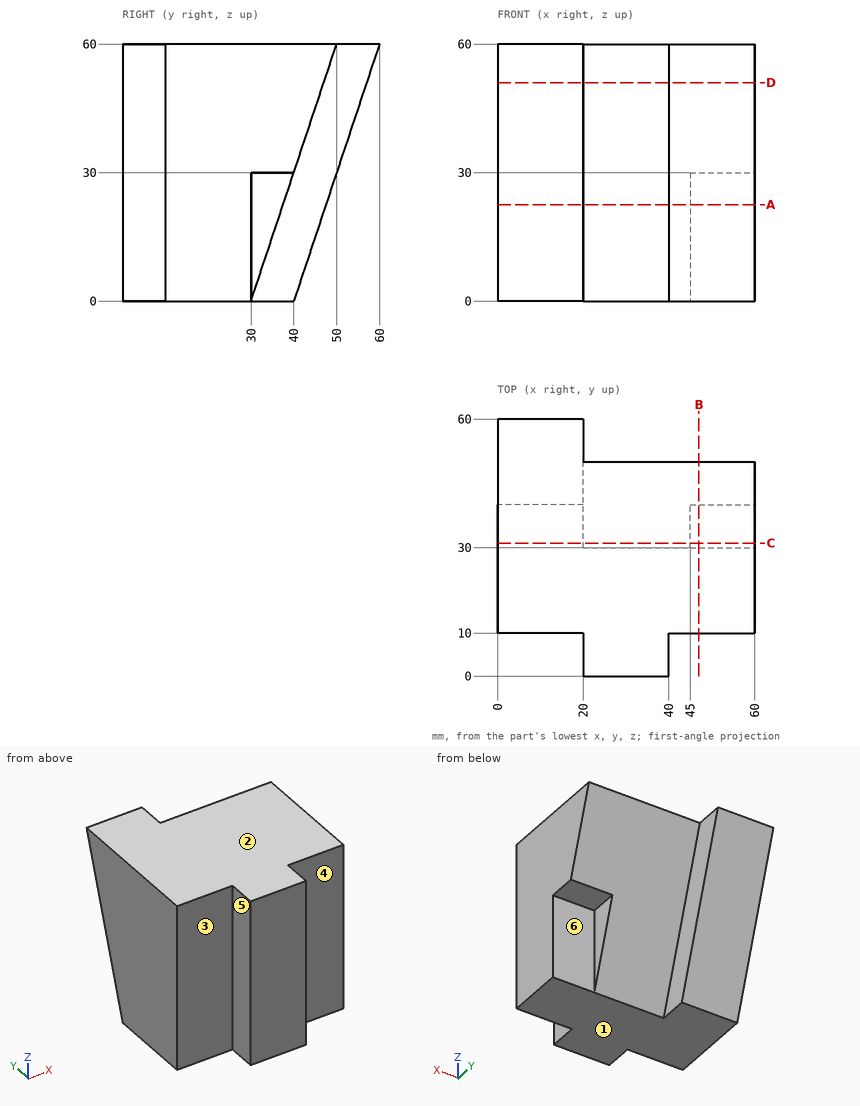
Design review of the part shown in the three views and the two pictorial views. Dimensions are in mm from the part's minimum x, y and z. A direction names the side the tool comes from. Coordinates: 2 decimals unless noted, no trailing zeros. Loops run counter-clockwise (first coordinate to the right, second up) from the corner with the lowest first, then second, coordinate; pieces in that order, holes last.
(1) Consider section C-C, the plane y = 31. Give the boundary of the cut face in (x, z).
Determined:
outline: (0, 0) - (20, 0) - (20, 3) - (45, 3) - (45, 30) - (60, 30) - (60, 60) - (0, 60) - close
(2) Draft analysis for pull direction Z (two halves, no side actions). For the marked faces 1, 2 and 3, state which applies: +Z half, -Z half, draft (parallel to the pull), parting line (faces both ways), or undercut.
Determined:
face 1: -Z half
face 2: +Z half
face 3: draft
(3) Insertion check: P1, Ø2, axis at x = 15.5, z = 26, coming from the -Y side; P2, Ø11, axis at y = 36, z = 12, coming from the +X side; P3, Ø9, axis at y = 46.5, z = 21, coming from the +X side. Each pin has a flat end and moves straight along its axis. Give the tip position at first contact, or say it passes through.
Determined:
P1: stops at y = 10
P2: stops at x = 45
P3: stops at x = 20
(4) Wall thickness on L1, parallel to Y at x = 58.5, z = 21.5; L2, parallel to X at y = 36.5, z = 15; L3, parallel to Y at x = 32.5, z = 46: over which ranges is each line inside the solid? List them lowest first.
Determined:
L1: y = 10 to 30
L2: x = 0 to 20
L3: y = 0 to 45.33
(5) Consider section B-B, the plane x = 47. Give the boundary of the cut face in (y, z), plus the area to 3 significant figures.
Determined:
outline: (10, 0) - (30, 0) - (30, 30) - (40, 30) - (50, 60) - (10, 60) - close
area: 1,650 mm2
(6) Consider section A-A, the plane z = 22.5. Give the boundary of the cut face in (x, y), plus the area to 3 significant figures.
Determined:
outline: (0, 10) - (20, 10) - (20, 0) - (40, 0) - (40, 10) - (60, 10) - (60, 30) - (45, 30) - (45, 37.5) - (20, 37.5) - (20, 47.5) - (0, 47.5) - close
area: 1,940 mm2
(7) Tool access review of the marked faces 4, 5 and 6: name each direction out of +Z, -Z, +X, -X, +Y, -Y from which nothing blocks a thin tool from reaching the whole face with its end or side.
Determined:
face 4: +Z, -Z, +X, -Y
face 5: +Z, -Z, -X, -Y
face 6: -Z, +X, +Y
(8) Consider section D-D, the plane z = 51. Give the boundary of the cut face in (x, y).
Determined:
outline: (0, 10) - (20, 10) - (20, 0) - (40, 0) - (40, 10) - (60, 10) - (60, 47) - (20, 47) - (20, 57) - (0, 57) - close
